from build123d import *

# Parameters (mm, degrees)
F0_W     = 50
F0_H     = 25
F1_DEPTH = 25
F2_R     = 5
F3_DEPTH = 25
F4_SIZE  = 1
F5_R     = 2.5
F6_DEPTH = 25


with BuildPart() as f1:
    # F0 (on Front) → F1 (new body)
    with BuildSketch(Plane.XZ):
        Rectangle(F0_W, F0_H)
    extrude(amount=F1_DEPTH)

    # F2 (on face) → F3 (cut)
    with BuildSketch(Plane.XZ.offset(25)):
        Circle(F2_R)
        with Locations((15, 0)):
            Circle(F2_R)
        with Locations((-15, 0)):
            Circle(F2_R)
    extrude(amount=-F3_DEPTH, mode=Mode.SUBTRACT)

    # F4
    f4_edges = [f1.edges().sort_by_distance(p)[0] for p in [
        (0, -25, -12.5),
        (-25, -25, 0),
        (25, -25, 0),
        (0, -25, 12.5),
        (-20, -25, 0),
        (-5, -25, 0),
        (10, -25, 0),
        (0, 0, -12.5),
        (-25, 0, 0),
        (25, 0, 0),
        (0, 0, 12.5),
        (-20, 0, 0),
        (-5, 0, 0),
        (10, 0, 0),
    ]]
    chamfer(f4_edges, length=F4_SIZE)

    # F5 (on face) → F6 (cut)
    with BuildSketch(Plane.XZ.offset(25)):
        with Locations((-24, 11.5)):
            Circle(F5_R)
        with Locations((24, 11.5)):
            Circle(F5_R)
        with Locations((24, -11.5)):
            Circle(F5_R)
        with Locations((-24, -11.5)):
            Circle(F5_R)
    extrude(amount=-F6_DEPTH, mode=Mode.SUBTRACT)


solid = f1.part
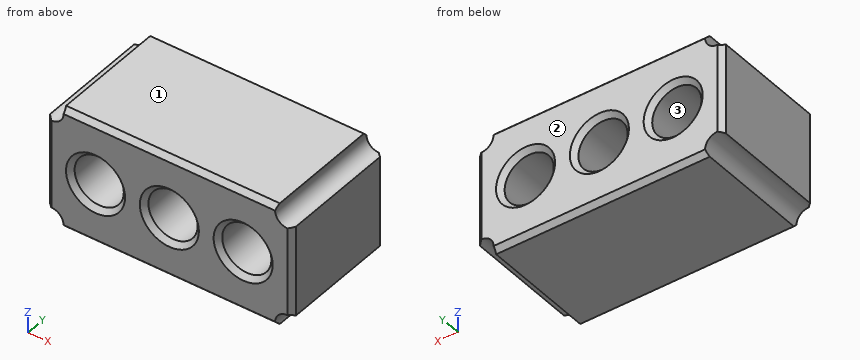
Can you work these out from the model? Positions are in its coordinate system, mm. Face numbers are marked on the shaded views. Round coordinates to 2 decimals unless told otherwise and drop trailing zeros. Loops run counter-clockwise (first coordinate to the right, second up) from the corner with the lowest first, then second, coordinate; pieces in that order, holes last. Notation, with made-up numbers: (78, 81.5) - (107, 81.5) arc R13 cw to (107, 100.5) - close; hole circle Ø3 at (-34.5, -27.5). An arc over 180 degrees is marked (long way). Answer in a Markdown table with one row per item. Add a question column.
Q1. I want a section at C-C on y = -16.25. List the corners of the cut face in (x, z) for me, and give its area (3 significant figures).
Q2. For pin 1 Ø8 at (x, z) = (-15, 0) entering from +Y; pin 2 Ø11.5 at (x, z) = (15, 0) entering from +Y, each with a flat end and sliding along its axis, tell me the tip position at first contact or that it passes through.
Q3. I need wall thicknesses on L1, parallel to Z at x = -15, y = -17.75; L2, parallel to X at y = -8.75, z = 1.75; L3, parallel to X at y = -4.5, z = 4.25. Which ranges of each line are inside material? Lowest first, please.
Q4. I want a section at B-B on x = 0. List the corners of the cut face in (y, z) for me.
Q5. I want a section at A-A on z = 0. Count the separate pieces of the cut face and the enclosed holes in it, and give its area (3 significant figures).
Q6. We'd pull the mould along Z, two halves only. Please class the marked faces 1, 2 and 3: pulls with the +Z half, pulls with the -Z half, needs draft (parallel to the pull), parting line crosses it, or undercut.
A:
| question | item | result |
|---|---|---|
| 1 | outline | (-25, -9.21) arc R2.5 cw to (-21.71, -12.5) - (21.71, -12.5) arc R2.5 cw to (25, -9.21) - (25, 9.21) arc R2.5 cw to (21.71, 12.5) - (-21.71, 12.5) arc R2.5 cw to (-25, 9.21) - close; hole circle Ø10 at (-15, 0); hole circle Ø10 at (0, 0); hole circle Ø10 at (15, 0) |
| 1 | area | 971 mm^2 |
| 2 | pin 1 | through |
| 2 | pin 2 | y = -0.25 |
| 3 | L1 | -12.5 to -5, 5 to 12.5 |
| 3 | L2 | -25 to -19.68, -10.32 to -4.68, 4.68 to 10.32, 19.68 to 25 |
| 3 | L3 | -25 to -17.63, -12.37 to -2.63, 2.63 to 12.37, 17.63 to 25 |
| 4 | outline | (-25, -11.5) - (-24, -12.5) - (-1, -12.5) - (0, -11.5) - (0, -6) - (-1, -5) - (-24, -5) - (-25, -6) - close; (-25, 6) - (-24, 5) - (-1, 5) - (0, 6) - (0, 11.5) - (-1, 12.5) - (-24, 12.5) - (-25, 11.5) - close |
| 5 | separate pieces | 4 |
| 5 | enclosed holes | 0 |
| 5 | area | 492 mm^2 |
| 6 | face 1 | pulls with the +Z half |
| 6 | face 2 | needs draft |
| 6 | face 3 | undercut |
